Autodesk Inventor part; units mm, degrees
ref_plane "YZ Plane" through (0, 0, 0) normal (1, 0, 0) x (0, 1, 0)
ref_plane "XZ Plane" through (0, 0, 0) normal (0, 1, 0) x (-1, 0, 0)
sketch "Sketch1" plane through (0, 0, 0) normal (0, 1, 0) x (-1, 0, 0)
  circle A0 centre (0, 0) radius 7.9375
  dimension "d35" = 15.875
extrude "Extrusion1" add sketch "Sketch1" along normal blind 48.26
hole "Hole1" at (0, 0, 0) direction (0, 1, 0) diameter 10.668 end through all
ref_plane "Work Plane1" through (0, 0, 7.9375) normal (0, 0, 1) x (1, 0, 0)
sketch "Sketch2" plane through (0, 0, 7.9375) normal (0, 0, 1) x (1, 0, 0)
  line L0 (-7.9375, 0) -> (-7.9375, 48.26)
  line L1 (-7.9375, 0) -> (7.9375, 0)
  point P0 (0, 0)
  point P1 (0, 40.64)
  dimension "d11" = 40.64
hole "Hole2" at (0, 40.64, 7.9375) direction (0, 0, -1) diameter 2.6416 depth 7.62 tip angle 118
properties part number "ToolHolderAdapter_v1" material "Aluminum 6061"
Geometry: final body of the model. Coordinates: model frame, mm. Coordinates: 2 decimals unless noted, no trailing zeros. Order: outer loops, then holes, each group sorted by start corner. A loop starts at its lowest first (then second) coordinate and runs counter-clockwise, first axis right, second up.
(1) Section query C-C (x = -4.75). Return the cut outline in (y, z), plus the area to 3 significant figures.
(2) Section query D-D (y = 11). Return the cut outline in (x, z) (1 decimal), plus the area to 3 significant figures.
(3) Material intervals for probe 1 along Y at (x, z) = (0, 6.8); probe 2 along Z at (x, y) = (0, 38); probe 3 along X at (y, z) = (16, 0.25), sorted ascending.
(4) Section query A-A (z = 0). Return the cut outline in (x, y).
(5) Section query B-B (x = 0). Return the cut outline in (y, z).
(6) Draft query along X for faces 1 (the face through (1.9, 0, -5.2)), 2 (the face through (-0.06, 41.96, 6.53)), 3 (the face through (1.72, 23.79, 7.75)). Return one class per face: pulls with the +X half, pulls with the -X half, needs draft (parallel to the pull), parting line crosses it, or undercut.
(7) First-contact query: pin 1 (2 mm diameter, centred on x = 4, y = 23.5, fed in from +Z); pin 2 (1.6 mm diameter, centred on x = 0, y = 40.64, fed in from +Z); pin 3 (2 mm diameter, centred on x = 1.5, z = 5, fed in from -Y); pin 4 (1 mm diameter, centred on y = 36.5, z = -3.5, fed in from +X). Flat tips, straight axial feed; report the tip coordinate or a pass-through.
Solution:
1. outline: (0, -6.36) - (48.26, -6.36) - (48.26, -2.43) - (0, -2.43) - close; (0, 2.43) - (48.26, 2.43) - (48.26, 6.36) - (0, 6.36) - close
1. area: 380 mm2
2. outline: circle Ø15.9 at (0, 0); hole circle Ø10.7 at (0, 0)
2. area: 109 mm2
3. probe 1: y = 0 to 39.32, 41.96 to 48.26
3. probe 2: z = -7.94 to -5.33, 5.33 to 7.94
3. probe 3: x = -7.93 to -5.33, 5.33 to 7.93
4. outline: (-7.94, 0) - (-5.33, 0) - (-5.33, 48.26) - (-7.94, 48.26) - close; (5.33, 0) - (7.94, 0) - (7.94, 48.26) - (5.33, 48.26) - close
5. outline: (0, -7.94) - (48.26, -7.94) - (48.26, -5.33) - (0, -5.33) - close; (0, 5.33) - (39.32, 5.33) - (39.32, 7.94) - (0, 7.94) - close; (41.96, 5.33) - (48.26, 5.33) - (48.26, 7.94) - (41.96, 7.94) - close
6. face 1: needs draft
6. face 2: undercut
6. face 3: parting line crosses it
7. pin 1: stops at z = 7.35
7. pin 2: stops at z = -5.27
7. pin 3: stops at y = 0
7. pin 4: stops at x = 7.35
